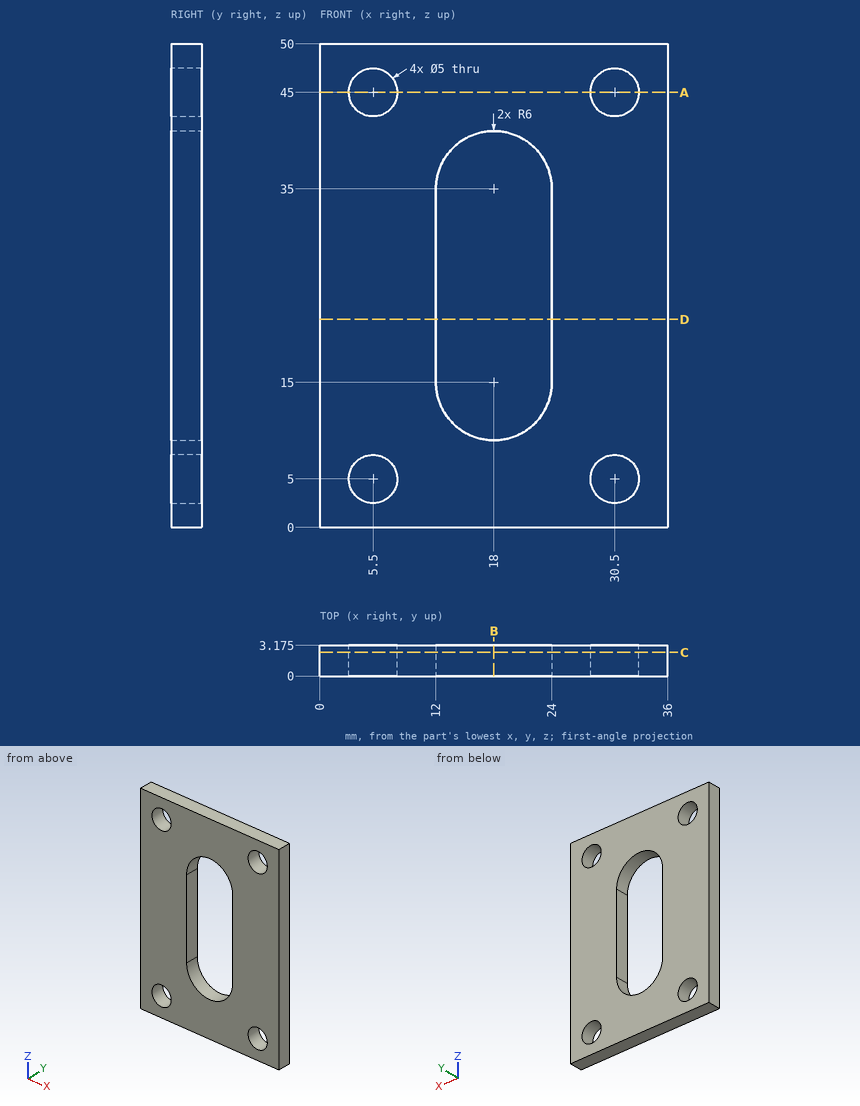
Input: dimensioned drawing with shaded views. Units: mm. Origin: part minimum x, y, z. Give positions to 0.01 mm unless a question says otherwise; leave off trailing zeros. Loops run counter-clockwise (first coordinate to the right, second up) from the corner with the lowest first, then second, coordinate; pieces in that order, holes last. Notation, with made-up numbers: M -30.75,61.5 L 0.25,61.5 A18 ccw 0.25,95.5 Z; hole C -6.75,3 d8. An arc over 180 degrees is marked long. Put each result on its own line as item: value.
1) First-contact query: P1, Ø6, axis at x = 30.5, z = 45, coming from the +Y side (3 decimals). Flat tip, straight axial feed; report the tip coordinate or a pass-through.
Computed values:
P1: stops at y = 3.175
2) Cut plane C-C, the plane y = 2.45. Return the cut outline in (x, z), plus the area to 3 significant figures.
Computed values:
outline: M 0,0 L 36,0 L 36,50 L 0,50 Z; hole C 5.5,5 d5; hole C 5.5,45 d5; hole M 12,15 A6 ccw 24,15 L 24,35 A6 ccw 12,35 Z; hole C 30.5,5 d5; hole C 30.5,45 d5
area: 1,370 mm^2
3) Cut plane A-A, the plane z = 45. Return the cut outline in (x, y) (3 decimals).
Computed values:
outline: M 0,0 L 3,0 L 3,3.175 L 0,3.175 Z; M 8,0 L 28,0 L 28,3.175 L 8,3.175 Z; M 33,0 L 36,0 L 36,3.175 L 33,3.175 Z
4) Cut plane D-D, the plane z = 21.5. Return the cut outline in (x, y) (3 decimals), plus the area to 3 significant figures.
Computed values:
outline: M 0,0 L 12,0 L 12,3.175 L 0,3.175 Z; M 24,0 L 36,0 L 36,3.175 L 24,3.175 Z
area: 76.2 mm^2
5) Material intervals for L1, parallel to X at y = 1.7, z = 45; L2, parallel to X at y = 1.65, z = 15; L3, parallel to Z at x = 6.5, y = 3.05, sorted ascending. Write a range as from..to.
Computed values:
L1: x = 0..3, 8..28, 33..36
L2: x = 0..12, 24..36
L3: z = 0..2.71, 7.29..42.71, 47.29..50
6) Cut plane B-B, the plane x = 18. Return the cut outline in (y, z) (3 decimals).
Computed values:
outline: M 0,0 L 3.175,0 L 3.175,9 L 0,9 Z; M 0,41 L 3.175,41 L 3.175,50 L 0,50 Z
